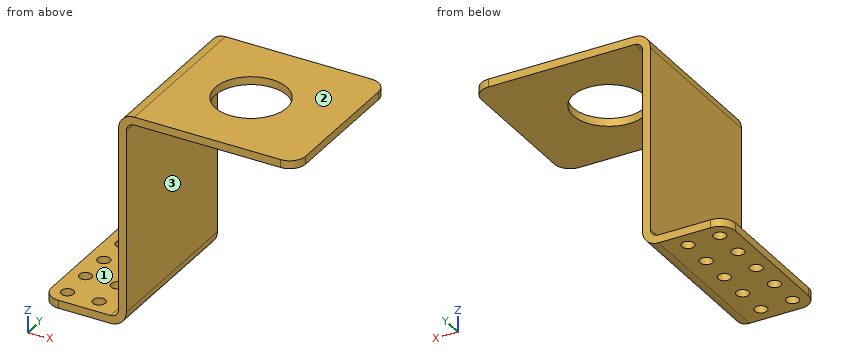
from build123d import *

# Parameters (mm, degrees)
SKETCH1_W           = 101.6
SKETCH1_H           = 63.5
BOSS_EXTRUDE1_DEPTH = 3.175
JOG1_DEPTH          = 63.5
JOG1_2_DEPTH        = 63.5
SKETCH7_R           = 14.2875
CUT_EXTRUDE1_DEPTH  = 146.496778315
SKETCH9_R           = 2.4892
CUT_EXTRUDE2_DEPTH  = 146.496778315
FILLET1_R           = 6.35


# Read off the part's stored shape, not the designer's step: Jog1
with BuildPart() as part:
    # Sketch1 → Boss-Extrude1 (new body)
    with BuildSketch(Plane.XY):
        with Locations((50.8, 31.75)):
            Rectangle(SKETCH1_W, SKETCH1_H)
    extrude(amount=BOSS_EXTRUDE1_DEPTH)

    # Jog1 outline → Jog1 (cut)
    with BuildSketch(Plane(origin=(0, 0, 0), x_dir=(1, 0, 0), z_dir=(0, 1, 0))):
        with BuildLine():
            ThreePointArc((27.247541247, 0), (30.422541247, -0.850738686), (32.746802561, -3.175))
            Line((32.746802561, -3.175), (101.6, -3.175))
            Line((101.6, -3.175), (101.6, 0))
            Line((101.6, 0), (27.247541247, 0))
        make_face()
    extrude(amount=JOG1_DEPTH, mode=Mode.SUBTRACT)

    # Jog1 2 outline → Jog1 2 (add)
    with BuildSketch(Plane(origin=(0, 0, 0), x_dir=(1, 0, 0), z_dir=(0, 1, 0))):
        with BuildLine():
            ThreePointArc((36.772541247, -82.55), (34.527477217, -81.62006403), (33.597541247, -79.375))
            Line((33.597541247, -79.375), (33.597541247, -6.35))
            ThreePointArc((33.597541247, -6.35), (33.381170244, -4.706499064), (32.746802561, -3.175))
            Line((32.746802561, -3.175), (27.247541247, -3.175))
            ThreePointArc((27.247541247, -3.175), (29.492605277, -4.10493597), (30.422541247, -6.35))
            Line((30.422541247, -6.35), (30.422541247, -79.375))
            ThreePointArc((30.422541247, -79.375), (32.282413186, -83.865128061), (36.772541247, -85.725))
            Line((36.772541247, -85.725), (101.6, -85.725))
            Line((101.6, -85.725), (101.6, -82.55))
            Line((101.6, -82.55), (36.772541247, -82.55))
        make_face()
    extrude(amount=JOG1_2_DEPTH)

    # Sketch7 → Cut-Extrude1 (cut, through all)
    with BuildSketch(Plane(origin=(0, 0, 82.55), x_dir=(-1, 0, 0), z_dir=(0, 0, -1))):
        with Locations(Location((-65.220541247, 31.75, 0), (0, 0, 90))):
            Circle(SKETCH7_R)
    extrude(amount=-CUT_EXTRUDE1_DEPTH, mode=Mode.SUBTRACT)

    # Sketch9 → Cut-Extrude2 (cut, through all)
    with BuildSketch(Plane.XY.offset(3.175)):
        with Locations((6.35, 57.15)):
            Circle(SKETCH9_R)
        with Locations(Location((19.05, 57.15, 0), (0, 0, 180))):
            Circle(SKETCH9_R)
        with Locations((6.35, 44.45)):
            Circle(SKETCH9_R)
        with Locations(Location((19.05, 44.45, 0), (0, 0, 180))):
            Circle(SKETCH9_R)
        with Locations((6.35, 31.75)):
            Circle(SKETCH9_R)
        with Locations(Location((19.05, 31.75, 0), (0, 0, 180))):
            Circle(SKETCH9_R)
        with Locations((6.35, 19.05)):
            Circle(SKETCH9_R)
        with Locations(Location((19.05, 19.05, 0), (0, 0, 180))):
            Circle(SKETCH9_R)
        with Locations((6.35, 6.35)):
            Circle(SKETCH9_R)
        with Locations(Location((19.05, 6.35, 0), (0, 0, 180))):
            Circle(SKETCH9_R)
    extrude(amount=-CUT_EXTRUDE2_DEPTH, mode=Mode.SUBTRACT)

    # Fillet1
    fillet1_edges = [part.edges().sort_by_distance(p)[0] for p in [
        (101.6, 63.5, 84.1375),
        (101.6, 0, 84.1375),
        (0, 0, 1.5875),
        (0, 63.5, 1.5875),
    ]]
    fillet(fillet1_edges, radius=FILLET1_R)


solid = part.part
Verification items for the finished model (mm, model axes). Face numbers are marked on the shaded views. A direction names the side the tool comes from. Give positions to 0.01 mm unless a question says otherwise; leave off trailing zeros. Loops run counter-clockwise (first coordinate to the right, second up) from the corner with the lowest first, then second, coordinate; pieces in that order, holes last.
1) Sectioned sample at C-C, the plane x = 75.5. Enter the section's corners in (y, z) (3 decimals), then the cut area to 3 significant figures.
2) Sectioned sample at B-B, the plane y = 19.05. Enter the section's corners in (x, z) (3 decimals), then the cut area to 3 significant figures.
3) Depth check by flat-ended pin: pin 1 Ø1 at (x, y) = (11, 45.5) entering from +Z (3 decimals); pin 2 Ø19 at (y, z) = (23.5, 45.5) entering from -X; pin 3 Ø19 at (y, z) = (26.5, 41.5) entering from +X. Enter the tip coordinate at first touch or a pass-through.
4) Sectioned sample at D-D, the plane z = 58. Enter the section's corners in (x, y).
5) Thickness scan on line 1 along Y through (x, z) = (6, 1); line 2 along X through (y, z) = (19, 2); line 3 along Z through (x, y) = (80.5, 4.5) (3 decimals). Record the ranges inside material, lowest first.
6) Set-up check for the marked faces 1, 2 and 3: record each of +Z, -Z, +X, -X, +Y, -Y from which the full face is reachable in a straight line by a thin tool's end or side.
7) Sectioned sample at A-A, the plane x = 19.05. Enter the section's corners in (y, z) (3 decimals).
Answers:
1. outline: (0, 82.55) - (21.827, 82.55) - (21.827, 85.725) - (0, 85.725) - close; (41.673, 82.55) - (63.5, 82.55) - (63.5, 85.725) - (41.673, 85.725) - close
1. area: 139 mm2
2. outline: (0, 0) - (3.861, 0) - (3.861, 3.175) - (0, 3.175) - close; (8.839, 0) - (16.561, 0) - (16.561, 3.175) - (8.839, 3.175) - close; (21.539, 0) - (27.248, 0) arc R6.35 ccw to (33.598, 6.35) - (33.598, 79.375) arc R3.175 cw to (36.773, 82.55) - (58.675, 82.55) - (58.675, 85.725) - (36.773, 85.725) arc R6.35 ccw to (30.423, 79.375) - (30.423, 6.35) arc R3.175 cw to (27.248, 3.175) - (21.539, 3.175) - close; (71.766, 82.55) - (101.6, 82.55) - (101.6, 85.725) - (71.766, 85.725) - close
2. area: 499 mm2
3. pin 1: stops at z = 3.175
3. pin 2: stops at x = 30.42
3. pin 3: stops at x = 33.6
4. outline: (30.42, 0) - (33.6, 0) - (33.6, 63.5) - (30.42, 63.5) - close
5. line 1: y = 0.01 to 3.89, 8.81 to 16.59, 21.51 to 29.29, 34.21 to 41.99, 46.91 to 54.69, 59.61 to 63.49
5. line 2: x = 0 to 3.86, 8.84 to 16.56, 21.54 to 31.87
5. line 3: z = 82.55 to 85.725
6. face 1: +Z, -X, +Y, -Y
6. face 2: +Z, +X, -X, +Y, -Y
6. face 3: -Z, +X, +Y, -Y
7. outline: (0, 0) - (3.861, 0) - (3.861, 3.175) - (0, 3.175) - close; (8.839, 0) - (16.561, 0) - (16.561, 3.175) - (8.839, 3.175) - close; (21.539, 0) - (29.261, 0) - (29.261, 3.175) - (21.539, 3.175) - close; (34.239, 0) - (41.961, 0) - (41.961, 3.175) - (34.239, 3.175) - close; (46.939, 0) - (54.661, 0) - (54.661, 3.175) - (46.939, 3.175) - close; (59.639, 0) - (63.5, 0) - (63.5, 3.175) - (59.639, 3.175) - close
